Autodesk Inventor part; units mm, degrees
ref_plane "YZ Plane" through (0, 0, 0) normal (1, 0, 0) x (0, 1, 0)
ref_plane "XZ Plane" through (0, 0, 0) normal (0, 1, 0) x (-1, 0, 0)
ref_plane "XY Plane" through (0, 0, 0) normal (0, 0, 1) x (1, 0, 0)
sketch "Sketch1" plane through (0, 0, 0) normal (0, 0, 1) x (1, 0, 0)
  line L0 (0, 0) -> (88.9, 0)
  line L1 (88.9, 0) -> (88.9, 31.75)
  line L2 (88.9, 31.75) -> (0, 31.75)
  line L3 (0, 31.75) -> (0, 0)
  circle A0 centre (12.7, 25.4) radius 3.302
  circle A1 centre (76.2, 25.4) radius 3.302
  circle A2 centre (12.7, 6.35) radius 3.302
  circle A3 centre (76.2, 6.35) radius 3.302
  line L4 (12.7, 25.4) -> (76.2, 25.4) construction
  line L5 (44.45, 31.75) -> (44.45, 0) construction
  point P0 (44.45, 25.4)
  dimension "d0" = 88.9
  dimension "d2" = 31.75
  dimension "d5" = 63.5
  dimension "d8" = 19.05
  dimension "d11" = 6.35
  dimension "d12" = 6.604
extrude "Extrusion1" add sketch "Sketch1" along normal blind 3.175
properties part number "M - Upper Rail Connector Plate 1" material "Aluminum 6061"
Source: CAD feature listing. Evaluate the final solid. Frame: model axes, mm. Round coordinates to 2 decimals unless told otherwise and drop trailing zeros. Loops run counter-clockwise (first coordinate to the right, second up) from the corner with the lowest first, then second, coordinate; pieces in that order, holes last. Notation, with made-up numbers: (-30.5, 9) - (-18.5, 9) arc R20 ccw to (-18.5, 23) - close; hole circle Ø11 at (42.5, 26.25). An arc over 180 degrees is marked (long way). Write item = value, one per line. Start each with the question number.
Item 1: Section query C-C on x = 76.2. Output: boundary loops of the cut face in (y, z) (3 decimals).
Item 2: Section query A-A on y = 25.4. Output: boundary loops of the cut face in (x, z) (3 decimals), plus the area to 3 significant figures.
Item 3: Mould query, pull axis X, two halves, no side actions, for faces 1 (the face through (44, 0, 2)), 2 (the face through (73.58, 27.41, 1.57)), 3 (the face through (0, 16, 2)). Classes: released by +X, released by -X, zero draft, split by the parting line, or undercut.
Item 4: Material intervals for line 1 (Y direction, x = 76.2, z = 2.5); line 2 (X direction, y = 23, z = 1.55); line 3 (Y direction, x = 77, z = 1.75), sorted ascending.
Item 5: First-contact query: pin 1 Ø4 at (x, y) = (12.7, 25.4) entering from +Z. Flat tip, straight axial feed; report the tip coordinate or a pass-through.
Item 6: Section query B-B on z = 2.45. Output: boundary loops of the cut face in (x, y), plus the area to 3 significant figures.
Results list:
q1.outline = (0, 0) - (3.048, 0) - (3.048, 3.175) - (0, 3.175) - close; (9.652, 0) - (22.098, 0) - (22.098, 3.175) - (9.652, 3.175) - close; (28.702, 0) - (31.75, 0) - (31.75, 3.175) - (28.702, 3.175) - close
q2.outline = (0, 0) - (9.398, 0) - (9.398, 3.175) - (0, 3.175) - close; (16.002, 0) - (72.898, 0) - (72.898, 3.175) - (16.002, 3.175) - close; (79.502, 0) - (88.9, 0) - (88.9, 3.175) - (79.502, 3.175) - close
q2.area = 240 mm²
q3.face_1 = zero draft
q3.face_2 = undercut
q3.face_3 = released by -X
q4.line_1 = 0 to 3.05, 9.65 to 22.1, 28.7 to 31.75
q4.line_2 = 0 to 10.43, 14.97 to 73.93, 78.47 to 88.9
q4.line_3 = 0 to 3.15, 9.55 to 22.2, 28.6 to 31.75
q5.pin_1 = through
q6.outline = (0, 0) - (88.9, 0) - (88.9, 31.75) - (0, 31.75) - close; hole circle Ø6.6 at (12.7, 6.35); hole circle Ø6.6 at (12.7, 25.4); hole circle Ø6.6 at (76.2, 6.35); hole circle Ø6.6 at (76.2, 25.4)
q6.area = 2,690 mm²
